```python
from build123d import *

# Parameters (mm, degrees)
BOSS_EXTRUDE1_DEPTH = 25.4
SKETCH2_R           = 2.921
CUT_EXTRUDE1_DEPTH  = 91.02678768
SKETCH3_W           = 4.7625
SKETCH3_H           = 50.8
CUT_EXTRUDE2_DEPTH  = 91.02678768
SKETCH4_W           = 44.45
SKETCH4_H           = 19.05
CUT_EXTRUDE3_DEPTH  = 91.02678768
FILLET1_R           = 5.08
SKETCH6_R           = 4.318
CUT_EXTRUDE5_DEPTH  = 12.7


with BuildPart() as part:
    # Sketch1 → Boss-Extrude1 (new body)
    with BuildSketch(Plane.XY):
        Polygon((0, 0), (0, 50.8), (25.4, 50.8), (25.4, 25.4), (69.85, 25.4), (69.85, 0), align=None)
    extrude(amount=BOSS_EXTRUDE1_DEPTH)

    # Sketch2 → Cut-Extrude1 (cut, through all)
    with BuildSketch(Plane.XY.offset(25.4)):
        with Locations((12.7, 38.1)):
            Circle(SKETCH2_R)
        with Locations((12.7, 12.7)):
            Circle(SKETCH2_R)
        with Locations((38.1, 12.7)):
            Circle(SKETCH2_R)
        with Locations((63.5, 12.7)):
            Circle(SKETCH2_R)
    extrude(amount=-CUT_EXTRUDE1_DEPTH, mode=Mode.SUBTRACT)

    # Sketch3 → Cut-Extrude2 (cut, through all)
    with BuildSketch(Plane.XY.offset(25.4)):
        with Locations((2.38125, 25.4)):
            Rectangle(SKETCH3_W, SKETCH3_H)
    extrude(amount=-CUT_EXTRUDE2_DEPTH, mode=Mode.SUBTRACT)

    # Sketch4 → Cut-Extrude3 (cut, through all)
    with BuildSketch(Plane.XZ):
        with Locations((47.625, 9.525)):
            Rectangle(SKETCH4_W, SKETCH4_H)
    extrude(amount=-CUT_EXTRUDE3_DEPTH, mode=Mode.SUBTRACT)

    # Fillet1
    fillet1_edges = [part.edges().sort_by_distance(p)[0] for p in [
        (25.4, 25.4, 22.225),
        (25.4, 12.7, 19.05),
    ]]
    fillet(fillet1_edges, radius=FILLET1_R)

    # Sketch6 → Cut-Extrude5 (cut)
    with BuildSketch(Plane.XY.offset(25.4)):
        with Locations((12.7, 38.1)):
            Circle(SKETCH6_R)
    extrude(amount=-CUT_EXTRUDE5_DEPTH, mode=Mode.SUBTRACT)


solid = part.part
```
Part model, mm, in its own coordinate system. A direction names the side the tool comes from. Round coordinates to 2 decimals unless told otherwise and drop trailing zeros. Loops run counter-clockwise (first coordinate to the right, second up) from the corner with the lowest first, then second, coordinate; pieces in that order, holes last.
1. Slice it at C-C (y = 12.7). Give the cut face in (x, z).
Solutions:
outline: (4.76, 0) - (9.78, 0) - (9.78, 25.4) - (4.76, 25.4) - close; (15.62, 0) - (25.4, 0) - (25.4, 13.97) arc R5.08 cw to (30.48, 19.05) - (35.18, 19.05) - (35.18, 25.4) - (15.62, 25.4) - close; (41.02, 19.05) - (60.58, 19.05) - (60.58, 25.4) - (41.02, 25.4) - close; (66.42, 19.05) - (69.85, 19.05) - (69.85, 25.4) - (66.42, 25.4) - close
2. Flat gauge pins, fed straight in: pin 1 (7.5 mm diameter, centred on y = 29, z = 9.5, fed in from +X); pin 2 (10 mm diameter, centred on x = 41.5, y = 11, fed in from -Z); pin 3 (1.9 mm diameter, centred on x = 42.5, z = 23, fed in from +Y). Where does each tip first touch, or does it go through?
Solutions:
pin 1: stops at x = 25.4
pin 2: stops at z = 19.05
pin 3: stops at y = 25.4
3. Drill centre lines: line 1 along Y through (x, z) = (12.7, 16); line 2 along Y through (x, z) = (12.7, 7.25); line 3 along Y through (x, z) = (38.1, 24). Where is each one in solid material? Low to high.
Solutions:
line 1: y = 0 to 9.78, 15.62 to 33.78, 42.42 to 50.8
line 2: y = 0 to 9.78, 15.62 to 35.18, 41.02 to 50.8
line 3: y = 0 to 9.78, 15.62 to 25.4
4. Two-plate mould, pull along Y, no slides. Class faces 1 (the face through (12.14, 42.38, 19.14)), 2 (the face through (23, 0, 15)), 3 (the face through (15, 50.8, 13)), 4 (the face through (15, 26, 0)): pulls with the +Y half, pulls with the -Y half, needs draft (parallel to the pull), parting line crosses it, or undercut.
Solutions:
face 1: undercut
face 2: pulls with the -Y half
face 3: pulls with the +Y half
face 4: needs draft
5. Slice it at A-A (x = 63.5). Give the cut face in (y, z).
Solutions:
outline: (0, 19.05) - (9.78, 19.05) - (9.78, 25.4) - (0, 25.4) - close; (15.62, 19.05) - (25.4, 19.05) - (25.4, 25.4) - (15.62, 25.4) - close
6. Slice it at B-B (x = 12.7). Give the cut face in (y, z).
Solutions:
outline: (0, 0) - (9.78, 0) - (9.78, 25.4) - (0, 25.4) - close; (15.62, 0) - (35.18, 0) - (35.18, 12.7) - (33.78, 12.7) - (33.78, 25.4) - (15.62, 25.4) - close; (41.02, 0) - (50.8, 0) - (50.8, 25.4) - (42.42, 25.4) - (42.42, 12.7) - (41.02, 12.7) - close
7. 3-axis set-ups, long thin cutter, end or side, ignore diameter. For faces 5 (the face through (16, 37, 12.7)), 6 (the face through (50, 25.4, 22)), 7 (the face through (50, 13, 19.05)), 8 (the face through (25.4, 31, 10)): which of +Z, -Z, +X, -X, +Y, -Y reach the whole face in a straight line?
Solutions:
face 5: +Z
face 6: +Z, -Z, +X, +Y
face 7: -Z, +X, +Y, -Y
face 8: -Z, +X, +Y
8. Slice it at D-D (z = 9). Give the cut face in (x, y), and give its area (3 significant figures).
Solutions:
outline: (4.76, 0) - (25.4, 0) - (25.4, 50.8) - (4.76, 50.8) - close; hole circle Ø5.84 at (12.7, 12.7); hole circle Ø5.84 at (12.7, 38.1)
area: 995 mm2
